For this review, take the finished solid that the model builds, in its own axes (mm). Round coordinates to 2 decimals unless told otherwise and drop trailing zeros. Write each loop counter-clockwise with the first axis right and the second up, starting at its lowest first coordinate (ties: lowest second). Pieces come first, ordered by that corner, then holes. Notation, with made-up numbers: (1.25, -40) -> (40.25, -40) arc R5 ccw to (40.25, -36) -> close; hole circle Ø8 at (53, 64). An arc over 180 degrees is marked (long way). Answer in a Markdown table with one row per item.
from build123d import *

# Parameters (mm, degrees)
BOSS_EXTRU_3_DEPTH            = 20
ENL_V_MAT_EXTRU_11_DEPTH      = 295.374154069
ENL_V_MAT_EXTRU_11_DEPTH_BACK = 249
ENL_V_MAT_EXTRU_12_DEPTH      = 295.374154069
ENL_V_MAT_EXTRU_12_DEPTH_BACK = 249
ENL_V_MAT_EXTRU_13_DEPTH      = 372.52143865
ENL_V_MAT_EXTRU_13_DEPTH_BACK = 249
ENL_V_MAT_EXTRU_14_DEPTH      = 372.52143865
ENL_V_MAT_EXTRU_14_DEPTH_BACK = 249
ENL_V_MAT_EXTRU_15_DEPTH      = 295.374154069
ENL_V_MAT_EXTRU_15_DEPTH_BACK = 249
ENL_V_MAT_EXTRU_16_DEPTH      = 295.374154069
ENL_V_MAT_EXTRU_16_DEPTH_BACK = 249
ENL_V_MAT_EXTRU_17_DEPTH      = 372.52143865
ENL_V_MAT_EXTRU_17_DEPTH_BACK = 249
ENL_V_MAT_EXTRU_18_DEPTH      = 372.52143865
ENL_V_MAT_EXTRU_18_DEPTH_BACK = 249
ESQUISSE17_R                  = 35
ENL_V_MAT_EXTRU_20_DEPTH      = 20


with BuildPart() as part:
    # Esquisse1 → Boss.-Extru.3 (new body)
    with BuildSketch(Plane.XY):
        Polygon((-263.060356118, 145.358531169), (-14.060356118, 145.358531169), (-14.060356118, 139.158531169), (-7.860356118, 139.158531169), (-7.860356118, -109.841468831), (-14.060356118, -109.841468831), (-14.060356118, -116.041468831), (-263.060356118, -116.041468831), (-263.060356118, -109.841468831), (-269.260356118, -109.841468831), (-269.260356118, 139.158531169), (-263.060356118, 139.158531169), align=None)
    extrude(amount=BOSS_EXTRU_3_DEPTH)

    # Esquisse4 → Enlèv. mat.-Extru.11 (cut, two sides: drawn at the far end of the back side and taken through both)
    with BuildSketch(Plane(origin=(-14.060356118, 0, 0), x_dir=(0, 0, -1), z_dir=(1, 0, 0)).offset(-ENL_V_MAT_EXTRU_11_DEPTH_BACK)):
        Polygon((-553.411816833, 139.158531169), (-20, 139.158531169), (-12.45, 139.158531169), (-12.45, 140.708531169), (-16.15, 140.708531169), (-16.15, 141.708531169), (-12.65, 145.358531169), (356.535030531, 530.365777294), (-64.826371106, 1510.451097334), (-974.77321847, 1119.243851209), align=None)
    extrude(amount=ENL_V_MAT_EXTRU_11_DEPTH + ENL_V_MAT_EXTRU_11_DEPTH_BACK, mode=Mode.SUBTRACT)

    # Esquisse8 → Enlèv. mat.-Extru.12 (cut, two sides: drawn at the far end of the back side and taken through both)
    with BuildSketch(Plane(origin=(-14.060356118, 0, 0), x_dir=(0, 0, -1), z_dir=(1, 0, 0)).offset(-ENL_V_MAT_EXTRU_12_DEPTH_BACK)):
        Polygon((533.411816833, 139.158531169), (0, 139.158531169), (-7.55, 139.158531169), (-7.55, 140.708531169), (-3.85, 140.708531169), (-3.85, 141.708531169), (-7.35, 145.358531169), (-376.535030531, 530.365777294), (44.826371106, 1510.451097334), (954.77321847, 1119.243851209), align=None)
    extrude(amount=ENL_V_MAT_EXTRU_12_DEPTH + ENL_V_MAT_EXTRU_12_DEPTH_BACK, mode=Mode.SUBTRACT)

    # Esquisse10 → Enlèv. mat.-Extru.13 (cut, two sides: drawn at the far end of the back side and taken through both)
    with BuildSketch(Plane(origin=(0, 139.158531169, 0), x_dir=(1, 0, 0), z_dir=(0, 1, 0)).offset(-ENL_V_MAT_EXTRU_13_DEPTH_BACK)):
        Polygon((-263.060356118, -20), (-263.060356118, -12.45), (-264.610356118, -12.45), (-264.610356118, -16.15), (-265.610356118, -16.15), (-269.260356118, -12.65), (-269.260356118, -20), align=None)
    extrude(amount=ENL_V_MAT_EXTRU_13_DEPTH + ENL_V_MAT_EXTRU_13_DEPTH_BACK, mode=Mode.SUBTRACT)

    # Esquisse11 → Enlèv. mat.-Extru.14 (cut, two sides: drawn at the far end of the back side and taken through both)
    with BuildSketch(Plane(origin=(0, 139.158531169, 0), x_dir=(1, 0, 0), z_dir=(0, 1, 0)).offset(-ENL_V_MAT_EXTRU_14_DEPTH_BACK)):
        Polygon((-643.553156031, -387.393505759), (-269.260356118, -7.35), (-265.813317082, -3.85), (-264.610356118, -3.85), (-264.610356118, -7.55), (-263.060356118, -7.55), (-263.060356118, 0), (-263.060356118, 533.411816833), (-1249.023765439, 940.82907325), (-1629.516565352, 20.023750658), align=None)
    extrude(amount=ENL_V_MAT_EXTRU_14_DEPTH + ENL_V_MAT_EXTRU_14_DEPTH_BACK, mode=Mode.SUBTRACT)

    # Esquisse12 → Enlèv. mat.-Extru.15 (cut, two sides: drawn at the far end of the back side and taken through both)
    with BuildSketch(Plane.ZY.offset(263.060356118).offset(-ENL_V_MAT_EXTRU_15_DEPTH_BACK)):
        Polygon((20, -109.841468831), (12.45, -109.841468831), (12.45, -111.391468831), (16.15, -111.391468831), (16.15, -112.391468831), (12.65, -116.041468831), (20, -116.041468831), align=None)
    extrude(amount=ENL_V_MAT_EXTRU_15_DEPTH + ENL_V_MAT_EXTRU_15_DEPTH_BACK, mode=Mode.SUBTRACT)

    # Esquisse13 → Enlèv. mat.-Extru.16 (cut, two sides: drawn at the far end of the back side and taken through both)
    with BuildSketch(Plane.ZY.offset(263.060356118).offset(-ENL_V_MAT_EXTRU_16_DEPTH_BACK)):
        Polygon((376.535030531, -501.048714956), (7.35, -116.041468831), (3.85, -112.391468831), (3.85, -111.391468831), (7.55, -111.391468831), (7.55, -109.841468831), (0, -109.841468831), (-533.411816833, -109.841468831), (-954.77321847, -1089.92678887), (-44.826371106, -1481.134034995), align=None)
    extrude(amount=ENL_V_MAT_EXTRU_16_DEPTH + ENL_V_MAT_EXTRU_16_DEPTH_BACK, mode=Mode.SUBTRACT)

    # Esquisse15 → Enlèv. mat.-Extru.17 (cut, two sides: drawn at the far end of the back side and taken through both)
    with BuildSketch(Plane(origin=(0, 139.158531169, 0), x_dir=(1, 0, 0), z_dir=(0, 1, 0)).offset(-ENL_V_MAT_EXTRU_17_DEPTH_BACK)):
        Polygon((-14.060356118, 0), (-14.060356118, -7.55), (-12.510356118, -7.55), (-12.510356118, -3.85), (-11.510356118, -3.85), (-7.860356118, -7.35), (-7.860356118, 0), align=None)
    extrude(amount=ENL_V_MAT_EXTRU_17_DEPTH + ENL_V_MAT_EXTRU_17_DEPTH_BACK, mode=Mode.SUBTRACT)

    # Esquisse16 → Enlèv. mat.-Extru.18 (cut, two sides: drawn at the far end of the back side and taken through both)
    with BuildSketch(Plane(origin=(0, 139.158531169, 0), x_dir=(1, 0, 0), z_dir=(0, 1, 0)).offset(-ENL_V_MAT_EXTRU_18_DEPTH_BACK)):
        Polygon((377.146890007, 356.535030531), (-7.860356118, -12.65), (-11.510356118, -16.15), (-12.510356118, -16.15), (-12.510356118, -12.45), (-14.060356118, -12.45), (-14.060356118, -20), (-14.060356118, -553.411816833), (966.024963922, -974.77321847), (1357.232210047, -64.826371106), align=None)
    extrude(amount=ENL_V_MAT_EXTRU_18_DEPTH + ENL_V_MAT_EXTRU_18_DEPTH_BACK, mode=Mode.SUBTRACT)

    # Esquisse17 → Enlèv. mat.-Extru.20 (cut)
    with BuildSketch(Plane(origin=(0, 0, 0), x_dir=(-1, 0, 0), z_dir=(0, 0, -1))):
        with Locations((138.560356118, 14.658531169)):
            Circle(ESQUISSE17_R)
    extrude(amount=-ENL_V_MAT_EXTRU_20_DEPTH, mode=Mode.SUBTRACT)


solid = part.part
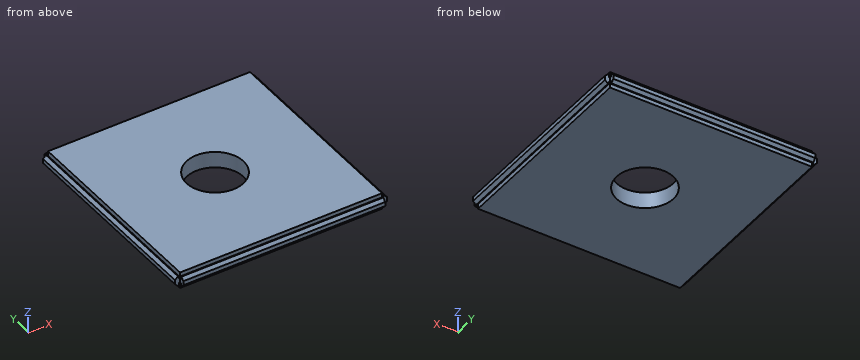
1) Consider section B-B on x = -24. State the section outline as (y, z) points, then the cut area to 3 significant figures.
Solved:
| item | result |
|---|---|
| outline | (-116.04, 7.35) -> (-112.39, 3.85) -> (-111.39, 3.85) -> (-111.39, 7.55) -> (-109.84, 7.55) -> (-109.84, 0) -> (139.16, 0) -> (139.16, 7.55) -> (140.71, 7.55) -> (140.71, 3.85) -> (141.71, 3.85) -> (145.36, 7.35) -> (145.36, 12.65) -> (141.71, 16.15) -> (140.71, 16.15) -> (140.71, 12.45) -> (139.16, 12.45) -> (139.16, 20) -> (-109.84, 20) -> (-109.84, 12.45) -> (-111.39, 12.45) -> (-111.39, 16.15) -> (-112.39, 16.15) -> (-116.04, 12.65) -> close |
| area | 5,080 mm² |
2) Consider section D-D on x = -116. State the section outline as (y, z) points.
Solved:
| item | result |
|---|---|
| outline | (-116.04, 7.35) -> (-112.39, 3.85) -> (-111.39, 3.85) -> (-111.39, 7.55) -> (-109.84, 7.55) -> (-109.84, 0) -> (-12.1, 0) -> (-12.1, 20) -> (-109.84, 20) -> (-109.84, 12.45) -> (-111.39, 12.45) -> (-111.39, 16.15) -> (-112.39, 16.15) -> (-116.04, 12.65) -> close; (41.42, 0) -> (139.16, 0) -> (139.16, 7.55) -> (140.71, 7.55) -> (140.71, 3.85) -> (141.71, 3.85) -> (145.36, 7.35) -> (145.36, 12.65) -> (141.71, 16.15) -> (140.71, 16.15) -> (140.71, 12.45) -> (139.16, 12.45) -> (139.16, 20) -> (41.42, 20) -> close |
3) Consider section A-A on y = -13. State the section outline as (x, z) points, then the cut area to 3 significant figures.
Solved:
| item | result |
|---|---|
| outline | (-269.26, 7.35) -> (-265.81, 3.85) -> (-264.61, 3.85) -> (-264.61, 7.55) -> (-263.06, 7.55) -> (-263.06, 0) -> (-160.01, 0) -> (-160.01, 20) -> (-263.06, 20) -> (-263.06, 12.45) -> (-264.61, 12.45) -> (-264.61, 16.15) -> (-265.61, 16.15) -> (-269.26, 12.65) -> close; (-117.11, 0) -> (-14.06, 0) -> (-14.06, 7.55) -> (-12.51, 7.55) -> (-12.51, 3.85) -> (-11.51, 3.85) -> (-7.86, 7.35) -> (-7.86, 12.65) -> (-11.51, 16.15) -> (-12.51, 16.15) -> (-12.51, 12.45) -> (-14.06, 12.45) -> (-14.06, 20) -> (-117.11, 20) -> close |
| area | 4,230 mm² |
4) Clearance check with flat-ended pins moving along their axes: pin 1 Ø1.8 at (y, z) = (9, 6) entering from +X; pin 2 Ø1.2 at (x, y) = (-13, 30) entering from +Z; pin 3 Ø1 at (x, z) = (-137.5, 5.5) entering from -Y. State where each tip first meets the part, or that it passes through.
Solved:
| item | result |
|---|---|
| pin 1 | x = -8.33 |
| pin 2 | z = 16.15 |
| pin 3 | y = -114.63 |
5) For line 1 (Y direction, x = -48.5, z = 7.5); line 2 (X direction, y = 109, z = 7.5); line 3 (X direction, y = 75, z = 15.5), list the stretches that pass through material, from the lowest coordinate up. Write a range as [from, to].
Solved:
| item | result |
|---|---|
| line 1 | [-116.04, -111.39], [-109.84, 139.16], [140.71, 145.36] |
| line 2 | [-269.26, -264.61], [-263.06, -14.06], [-12.51, -7.86] |
| line 3 | [-266.29, -264.61], [-263.06, -14.06], [-12.51, -10.83] |
6) Consider section C-C on y = -83.5. State the section outline as (x, z) points.
Solved:
| item | result |
|---|---|
| outline | (-269.26, 7.35) -> (-265.81, 3.85) -> (-264.61, 3.85) -> (-264.61, 7.55) -> (-263.06, 7.55) -> (-263.06, 0) -> (-14.06, 0) -> (-14.06, 7.55) -> (-12.51, 7.55) -> (-12.51, 3.85) -> (-11.51, 3.85) -> (-7.86, 7.35) -> (-7.86, 12.65) -> (-11.51, 16.15) -> (-12.51, 16.15) -> (-12.51, 12.45) -> (-14.06, 12.45) -> (-14.06, 20) -> (-263.06, 20) -> (-263.06, 12.45) -> (-264.61, 12.45) -> (-264.61, 16.15) -> (-265.61, 16.15) -> (-269.26, 12.65) -> close |
